Part model, mm, in its own coordinate system. Give positions to 0.01 mm unless a question says otherwise; leave off trailing zeros. Loops run counter-clockwise (first coordinate to the right, second up) from the corner with the lowest first, then second, coordinate; pieces in that order, holes last. Notation, with made-up numbers: M 23.25,54.25 L 58.25,54.25 A22 ccw 58.25,79.25 Z; hole C -10.75,46 d8. An arc over 180 degrees is marked long. Put each result on its own line as item: value. Start each with the question number.
Autodesk Inventor part; units mm, degrees
ref_plane "Start Plane" through (0, 0, -2.5822) normal (0, 0, 1) x (1, 0, 0)
ref_plane "End Plane" through (0, 0, 69.1479) normal (0, 0, 1) x (1, 0, 0)
ref_plane "Work Plane4" through (6.5224, 8.4418, 69.2424) normal (-0.0922, -0.1193, 0.9886) x (0.9957, -0.0055, 0.0922)
ref_plane "Start Plane" through (0, 0, -2.5822) normal (0, 0, 1) x (1, 0, 0)
ref_plane "End Plane" through (0, 0, 69.1479) normal (0, 0, 1) x (1, 0, 0)
sketch "Sketch" plane through (0, 0, 0) normal (0, 0, 1) x (1, 0, 0)
  circle A0 centre (0, 0) radius 6.9342
  circle A1 centre (0, 0) radius 10.668
  dimension "d0" = 21.336
  dimension "d1" = 3.7338
extrude "Body" add sketch "Sketch" along normal up to surface (71.7301 mm away) from surface at -2.5822
sketch "Sketch3" plane through (0, 0, 0) normal (0, 0, 1) x (1, 0, 0)
  line L0 (0, 0) -> (10, 0)
ref_plane "Work Plane3" through (0, 0, 0) normal (0, -1, 0) x (1, 0, 0)
sketch "Sketch4" plane through (0, 0, 0) normal (0, -1, 0) x (1, 0, 0)
  line L0 (-2, -2.5822) -> (12, -2.5822)
  line L1 (-2, 69.1479) -> (12, 69.1479)
  dimension "d7" = 71.7301
ref_plane "Work Plane4" through (6.5224, 8.4418, 69.2424) normal (-0.0922, -0.1193, 0.9886) x (0.9957, -0.0055, 0.0922)
split "Split1" plane through (6.5224, 8.4418, 69.2424) removes the side toward (-0.0922, -0.1193, 0.9886)
ref_plane "Work Plane5" through (0, 10.668, -2.5822) normal (0, -0.2353, -0.9719) x (1, 0, 0)
split "Split2" plane through (0, 10.668, -2.5822) removes the side toward (0, -0.2353, -0.9719)
ref_plane "Work Plane6" through (-10.3791, 2.4658, -9.228) normal (0.6365, -0.1512, -0.7563) x (-0.6625, 0.395, -0.6365)
split "Split3" plane through (-10.3791, 2.4658, -9.228) removes the side toward (0.6365, -0.1512, -0.7563)
ref_plane "Work Plane7" through (-9.0379, 5.6677, 73.9403) normal (0.432, -0.2709, 0.8602) x (0.8997, 0.0629, -0.432)
split "Split4" plane through (-9.0379, 5.6677, 73.9403) removes the side toward (0.432, -0.2709, 0.8602)
equation "\"d0\" = G_H"
equation "\"d1\" = G_T"
equation "\"d2\" = G_L"
equation "\"G_H\" = 21.336"
equation "\"G_T\" = 3.7338"
equation "\"G_L\" = 71.72685"
equation "\"G_OFFSET_START\" = 2.58216"
equation "\"G_OFFSET_END\" = 1.53222"
equation "\"d4\" = -G_OFFSET_START"
equation "\"d5\" = G_OFFSET_END + B_L"
equation "\"B_L\" = 67.6157"
properties part number "ANSI - 1/2 x 0.147 - 2.824" material "Steel, Mild"
1) Wall check: L1, parallel to X at y = 0, z = 13.5; L2, parallel to X at y = -5.25, z = 40.5. Give the ranges that are in metal, low to high.
2) Band-saw the part on A-A on x = 1.5. Give the cut face in (y, z).
3) Band-saw the part on D-D on x = 9.25. Give the cut face in (y, z).
4) Band-saw the part on C-C on z = 24. Give the cut face in (x, y).
5) Band-saw the part on B-B on y = -4.5. Give the cut face in (x, z), then the cut area to 3 significant figures.
6) Mould opens along Y. For faces 1 (the cylindrical face through (-8.466, 6.491, 32.782)), 2 (the flat face through (6.69, -4.28, 62.91)), 3 (the cylindrical face through (-5.5, 4.22, 32.98)) say: +Y half, -Y half, draft (parallel to the pull), parting line (faces both ways), or undercut.
7) Pin check, flat tips, straight feed: pin 1 Ø5 at (x, z) = (-8, 47) entering from -Y; pin 2 Ø1 at (x, y) = (-7, -1) entering from +Z; pin 3 Ø12 at (x, y) = (3.5, 6) entering from -Z. Stop position of each tip, or through.
Evaluation:
1. L1: -10.67 to -6.93, 6.93 to 10.67
1. L2: -9.29 to -4.53, 4.53 to 9.29
2. outline: M -10.56,3.37 L -6.77,2.62 L -6.77,64.73 L -10.56,63.54 Z; M 6.77,-0.09 L 10.56,-0.85 L 10.56,69.03 L 6.77,68.57 Z
3. outline: M -5.31,8.85 L 5.31,6.72 L 5.31,64.64 L -5.31,61.3 Z
4. outline: C 0,0 d21.34; hole C 0,0 d13.87
5. outline: M -9.67,1.09 L -5.28,1.09 L -5.28,66.58 L -9.67,66.17 Z; M 5.28,5.34 L 9.67,9.04 L 9.67,61.34 L 5.28,63.55 Z
5. area: 530 mm2
6. face 1: parting line
6. face 2: -Y half
6. face 3: undercut
7. pin 1: y = -9.14
7. pin 2: z = 66.91
7. pin 3: z = -2.53
